Design review of the part shown in the three views and the two pictorial views. Dimensions are in mm from the part's minimum x, y and z. A direction names the side the tool comes from. Round coordinates to 2 decimals unless told otherwise and drop trailing zeros. Loops run counter-clockwise (first coordinate to the right, second up) from the corner with the lowest first, then second, coordinate; pieces in that order, holes last. Notation, with made-up numbers: M -24.75,31.25 L 11.25,31.25 A22 ccw 11.25,64.25 Z; hole C -33,-15.75 d6. An arc over 180 degrees is marked long. Return JSON: item names as keys, results as strings. Group by question number.
Q1. Clearance check with flat-ended pins moving along their axes: pin 1 Ø9.5 at (y, z) = (4.5, 31) entering from +X; pin 2 Ø6 at (x, z) = (61.5, 19.5) entering from +Y; pin 3 Ø1 at (x, y) = (62.5, 38) entering from -Z; pin 4 Ø1 at (x, y) = (91, 15.5) entering from +Z. State where each tip first meets the part, or that it passes through.
Q2. For the marked faces 1, 2 and 3, list the 3-axis set-ups (+Z, -Z, +X, -X, +Y, -Y) from which the entire face can be reached by the end or side of a thin tool; tool diameter is ignored.
Q3. Consider section A-A (x = 24). State the section outline as (y, z) points.
Q4. Consider section B-B (y = 8). State the section outline as (x, z) points.
Q5. Draft analysis for pull direction Y (two halves, no side actions). For the marked faces 4, 5 and 6, state which applies: pulls with the +Y half, pulls with the -Y half, needs draft (parallel to the pull), parting line crosses it, or undercut.
Q6. To check wall thickness, follow line 1 along Y through (x, z) = (19.5, 59); line 2 along X through (y, z) = (39, 40); line 3 along Z through (x, y) = (12, 13.5). State the ranges of each line that lie inside material, in increasing order.
Q7. Consider section C-C (z = 57.5). State the section outline as (x, y) points, and give its area (3 significant figures).
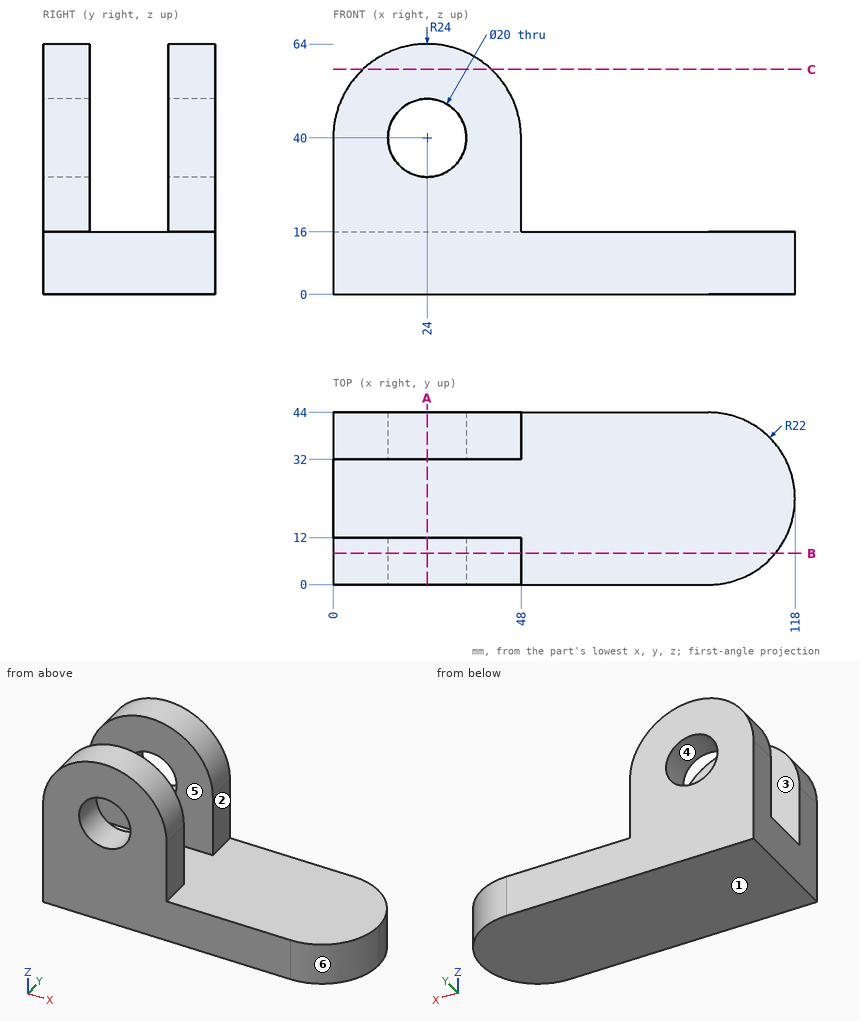
Values:
{
 "1": {"pin 1": "stops at x = 48", "pin 2": "passes through", "pin 3": "stops at z = 0", "pin 4": "stops at z = 16"},
 "2": {"face 1": "-Z, +X, -X, +Y, -Y", "face 2": "+Z, +X, +Y, -Y", "face 3": "+Z, +X, -X"},
 "3": {"outline": "M 0,0 L 44,0 L 44,30 L 32,30 L 32,16 L 12,16 L 12,30 L 0,30 Z; M 0,50 L 12,50 L 12,64 L 0,64 Z; M 32,50 L 44,50 L 44,64 L 32,64 Z"},
 "4": {"outline": "M 0,0 L 112.97,0 L 112.97,16 L 48,16 L 48,40 A24 ccw 0,40 Z; hole C 24,40 d20"},
 "5": {"face 4": "needs draft", "face 5": "undercut", "face 6": "pulls with the -Y half"},
 "6": {"line 1": "y = 0 to 12, 32 to 44", "line 2": "x = 0 to 14, 34 to 48", "line 3": "z = 0 to 16"},
 "7": {"outline": "M 7.58,0 L 40.42,0 L 40.42,12 L 7.58,12 Z; M 7.58,32 L 40.42,32 L 40.42,44 L 7.58,44 Z", "area": "788 mm2"}
}
